CAD build for the part. Positions are in the model's coordinates, mm. Coordinates: 2 decimals unless noted, no trailing zeros. Loops run counter-clockwise (first coordinate to the right, second up) from the corner with the lowest first, then second, coordinate; pieces in that order, holes last. Notation, with made-up numbers: (40.25, 40) -> (89.25, 40) arc R36 cw to (89.25, 77) -> close; hole circle Ø5 at (-17.75, -25). An arc over 180 degrees is marked (long way). Write item = value, one per line. Start each with the question number.
(1) Flat gauge pin, fed straight in: P1, Ø8, axis at x = 50.8, y = 9.525, coming from the +Z side. Where does the tip first touch, or does it go through?
(2) Drill centre lines: line 1 (X direction, y = 10, z = 1.4); line 2 (X direction, y = 6.25, z = 1.6); line 3 (Y direction, x = 114.3, z = 1.45). Where is each one in solid material? Low to high. Write a range as from..to.
(3) Band-saw the part on A-A (z = 1.9). Write the cut outline in (x, y) (3 decimals).
```python
from build123d import *

# Parameters (mm, degrees)
SKETCH1_W           = 558.8
SKETCH1_H           = 19.05
BOSS_EXTRUDE1_DEPTH = 4.7752
SKETCH2_R           = 3.5687
CUT_EXTRUDE1_DEPTH  = 560.145012528


with BuildPart() as part:
    # Sketch1 → Boss-Extrude1 (new body)
    with BuildSketch(Plane.XY):
        with Locations((279.4, 9.525)):
            Rectangle(SKETCH1_W, SKETCH1_H)
    extrude(amount=BOSS_EXTRUDE1_DEPTH)

    # Sketch2 → Cut-Extrude1 (cut, through all)
    with BuildSketch(Plane.XY):
        with Locations((50.8, 9.525)):
            Circle(SKETCH2_R)
        with Locations((114.3, 9.525)):
            Circle(SKETCH2_R)
        with Locations((228.6, 9.525)):
            Circle(SKETCH2_R)
        with Locations((342.9, 9.525)):
            Circle(SKETCH2_R)
        with Locations((457.2, 9.525)):
            Circle(SKETCH2_R)
    extrude(amount=CUT_EXTRUDE1_DEPTH, mode=Mode.SUBTRACT)


solid = part.part
```
Findings below:
q1.P1 = 4.78
q2.line_1 = 0..47.26, 54.34..110.76, 117.84..225.06, 232.14..339.36, 346.44..453.66, 460.74..558.8
q2.line_2 = 0..49.38, 52.22..112.88, 115.72..227.18, 230.02..341.48, 344.32..455.78, 458.62..558.8
q2.line_3 = 0..5.96, 13.09..19.05
q3.outline = (0, 0) -> (558.8, 0) -> (558.8, 19.05) -> (0, 19.05) -> close; hole circle Ø7.137 at (50.8, 9.525); hole circle Ø7.137 at (114.3, 9.525); hole circle Ø7.137 at (228.6, 9.525); hole circle Ø7.137 at (342.9, 9.525); hole circle Ø7.137 at (457.2, 9.525)
